Source: CAD feature listing. Evaluate the final solid. Frame: model axes, mm. A direction names the side the tool comes from. Give positions to 0.01 mm unless a question says otherwise; leave off trailing zeros. Order: outer loops, then holes, each group sorted by start corner. A loop starts at its lowest first (then second) coordinate and runs counter-clockwise, first axis right, second up. Notation, with made-up numbers: M 25.25,26.5 L 60.25,26.5 A21 cw 60.25,48.5 Z; hole C -7.75,-32.75 d11. An arc over 180 degrees is marked long. Answer as a JSON object with one key per item and string values. Group by question number.
1. Pull-direction query (Z, two-part tool) for faces 4 (the flat face through (-19, 63, 0.5)), 5 (the cylindrical face through (0.16, 12.5, -0.05)), 6 (the cylindrical face through (12.55, 1.48, -0.07)); classes: +Z half, -Z half, draft (parallel to the pull), parting line (faces both ways), or undercut.
2. Section query A-A (y = 95). Output: boundary loops of the cut face in (x, z), plus the area to 3 significant figures.
3. Section query B-B (x = -11). Output: boundary loops of the cut face in (y, z).
4. Section query C-C (x = 6). Output: boundary loops of the cut face in (y, z), plus the area to 3 significant figures.
5. Material intervals for L1, parallel to Z at x = -11, y = 0.7; L2, parallel to Y at x = 5.5, z = -2.75; L3, parallel to X at y = 65, z = 1.2, sorted ascending. Write a range as [from, to].
6. Set-up query: faces 1 (the cylindrical face through (17.79, 68.57, -1.53)), 2 (the flat face through (0, 0, 0)), 3 (the flat face through (-11, 9, 0)). Return all of +Z, -Z, +X, -X, +Y, -Y with unobstructed straight access to the full face (end or side cutting, diameter ignored); none if empty.
7. Section query D-D (y = 75). Output: boundary loops of the cut face in (x, z) (3 decimals), plus the area to 3 significant figures.
8. Pin query (flat end, axial travel): P1, Ø1.8, axis at x = 12, z = 1, coming from the +Y side; P2, Ø1.5, axis at y = 51.5, z = 0, coming from the +X side; P3, Ø4, axis at x = 15, z = -1.5, coming from the +Y side. Return the tip coordinate at first contact, or that it passes through.
from build123d import *

# Parameters (mm, degrees)
SKETCH_1_R         = 2.05
SKETCH_1_R_2       = 10
EXTRUDE_1_DEPTH    = 3.5
SKETCH1_R          = 12.025
CUT_EXTRUDE2_DEPTH = 5
SKETCH3_R          = 3.6
CUT_EXTRUDE4_DEPTH = 4
SKETCH4_R          = 1.55
CUT_EXTRUDE5_DEPTH = 5


with BuildPart() as part:
    # 草图1 → 凸台-拉伸1 (new, symmetric)
    with BuildSketch(Plane.XY):
        with BuildLine():
            Line((-19, 0), (19, 0))
            Line((19, 0), (19, 57))
            ThreePointArc((19, 57), (19.25658351, 58.58113883), (20, 60))
            ThreePointArc((20, 60), (0, 100), (-20, 60))
            ThreePointArc((-20, 60), (-19.25658351, 58.58113883), (-19, 57))
            Line((-19, 57), (-19, 0))
        make_face()
        with BuildLine():
            Line((7.5, 45), (7.5, 20))
            ThreePointArc((7.5, 20), (0, 12.5), (-7.5, 20))
            Line((-7.5, 20), (-7.5, 45))
            ThreePointArc((-7.5, 45), (-5.303300859, 50.303300859), (0, 52.5))
            ThreePointArc((0, 52.5), (5.303300859, 50.303300859), (7.5, 45))
        make_face(mode=Mode.SUBTRACT)
        with BuildLine():
            ThreePointArc((-8, 9), (-5, 6), (-8, 3))
            Line((-8, 3), (-14, 3))
            ThreePointArc((-14, 3), (-17, 6), (-14, 9))
            Line((-14, 9), (-8, 9))
        make_face(mode=Mode.SUBTRACT)
        with BuildLine():
            ThreePointArc((8, 3), (5, 6), (8, 9))
            Line((8, 9), (14, 9))
            ThreePointArc((14, 9), (17, 6), (14, 3))
            Line((14, 3), (8, 3))
        make_face(mode=Mode.SUBTRACT)
        with Locations((0, 95)):
            Circle(SKETCH_1_R, mode=Mode.SUBTRACT)
        with Locations((-17.320508076, 65)):
            Circle(SKETCH_1_R, mode=Mode.SUBTRACT)
        with Locations((0, 75)):
            Circle(SKETCH_1_R_2, mode=Mode.SUBTRACT)
        with Locations((17.320508076, 65)):
            Circle(SKETCH_1_R, mode=Mode.SUBTRACT)
    extrude(amount=EXTRUDE_1_DEPTH, both=True)

    # Sketch1 → Cut-Extrude2 (cut)
    with BuildSketch(Plane(origin=(0, 0, -3.5), x_dir=(-1, 0, 0), z_dir=(0, 0, -1))):
        with Locations((0, 75)):
            Circle(SKETCH1_R)
    extrude(amount=-CUT_EXTRUDE2_DEPTH, mode=Mode.SUBTRACT)

    # Sketch3 → Cut-Extrude4 (cut)
    with BuildSketch(Plane(origin=(0, 0, -3.5), x_dir=(-1, 0, 0), z_dir=(0, 0, -1))):
        with Locations((0, 95)):
            Circle(SKETCH3_R)
        with Locations((17.320508076, 65)):
            Circle(SKETCH3_R)
        with Locations((-17.320508076, 65)):
            Circle(SKETCH3_R)
    extrude(amount=-CUT_EXTRUDE4_DEPTH, mode=Mode.SUBTRACT)

    # Sketch4 → Cut-Extrude5 (cut)
    with BuildSketch(Plane(origin=(0, 0, 0), x_dir=(-1, 0, 0), z_dir=(0, -1, 0))):
        with Locations(Location((11, 0, 0), (0, 0, 180))):
            Circle(SKETCH4_R)
        with Locations((-11, 0)):
            Circle(SKETCH4_R)
    extrude(amount=-CUT_EXTRUDE5_DEPTH, mode=Mode.SUBTRACT)


solid = part.part
Answer sheet:
{
 "1": {"face 4": "-Z half", "face 5": "draft", "face 6": "undercut"},
 "2": {"outline": "M -15,-3.5 L -3.6,-3.5 L -3.6,0.5 L -2.05,0.5 L -2.05,3.5 L -15,3.5 Z; M 2.05,0.5 L 3.6,0.5 L 3.6,-3.5 L 15,-3.5 L 15,3.5 L 2.05,3.5 Z", "area": "169 mm^2"},
 "3": {"outline": "M 0,-3.5 L 3,-3.5 L 3,-1.55 L 0,-1.55 Z; M 0,1.55 L 3,1.55 L 3,3.5 L 0,3.5 Z; M 9,-3.5 L 70.14,-3.5 L 70.14,1.5 L 79.86,1.5 L 79.86,-3.5 L 97.45,-3.5 L 97.45,3.5 L 9,3.5 Z"},
 "4": {"outline": "M 0,-3.5 L 3.76,-3.5 L 3.76,3.5 L 0,3.5 Z; M 8.24,-3.5 L 15.5,-3.5 L 15.5,3.5 L 8.24,3.5 Z; M 49.5,-3.5 L 64.58,-3.5 L 64.58,1.5 L 67,1.5 L 67,3.5 L 49.5,3.5 Z; M 83,1.5 L 85.42,1.5 L 85.42,-3.5 L 99.27,-3.5 L 99.27,3.5 L 83,3.5 Z", "area": "289 mm^2"},
 "5": {"L1": "[-3.5, -1.55], [1.55, 3.5]", "L2": "[0, 4.34], [7.66, 14.9], [50.1, 64.31], [85.69, 99.39]", "L3": "[-22.91, -19.37], [-15.27, -6.68], [6.68, 15.27], [19.37, 22.91]"},
 "6": {"face 1": "-Z", "face 2": "+Z, -Z, +X, -X, -Y", "face 3": "+Z, -Z"},
 "7": {"outline": "M -25,-3.5 L -12.025,-3.5 L -12.025,1.5 L -10,1.5 L -10,3.5 L -25,3.5 Z; M 10,1.5 L 12.025,1.5 L 12.025,-3.5 L 25,-3.5 L 25,3.5 L 10,3.5 Z", "area": "190 mm^2"},
 "8": {"P1": "y = 97.4", "P2": "x = 19", "P3": "y = 96.35"}
}
